Design review of the part built by this model. Coordinates are the model's own, in mm. A direction names the side the tool comes from. Round coordinates to 2 decimals unless told otherwise and drop trailing zeros. Loops run counter-clockwise (first coordinate to the right, second up) from the corner with the lowest first, then second, coordinate; pieces in that order, holes last. Notation, with made-up numbers: M 48,52 L 81,52 A21 ccw 81,74 Z; hole C 63.25,-10.75 d10. An arc over 180 degrees is marked long. One line per item, written item: value. Start each with the question number.
Item 1: For line 1 along Y through (x, z) = (0, 1.3); line 2 along Y through (x, z) = (-8, 1); line 3 along Y through (x, z) = (12.5, 0.7), list the stretches that pass through material, from the lowest coordinate up.
Item 2: For faces 1 (the flat face through (-2.5, 0, 1)), 2 (the flat face through (15, 0, 1)), list the 3-axis set-ups (+Z, -Z, +X, -X, +Y, -Y) from which the entire face can be reached by the end or side of a thin tool; tool diameter is ignored.
Item 3: We need section B-B (x = 8). Write out the cut boundary in (y, z), then the cut area to 3 significant figures.
Item 4: We need section D-D (x = 13). Write out the cut boundary in (y, z), then the cut area to 3 significant figures.
Item 5: We need section A-A (y = -2.5). Write out the cut boundary in (x, z).
Item 6: We need section C-C (z = 1.5). Write out the cut boundary in (x, y).
Item 7: Mouldability with a two-part tool opening along Y and no side actions: class faces 3 (the flat face through (-15, 0, 1)), 4 (the cylindrical face through (11.763, -10.824, 1.014)), 5 (the cylindrical face through (14.1, -13.14, 1.01)) as released by +Y, released by -Y, zero draft, split by the parting line, or undercut.
from build123d import *

# Parameters (mm, degrees)
SKETCH_1_W          = 30
SKETCH_1_H          = 28
EXTRUDE_1_DEPTH     = 2
FILLET_1_R          = 3
SKETCH_2_R          = 1
SKETCH_2_R_2        = 1.25
CUT_EXTRUDE_1_DEPTH = 10
SKETCH_3_R          = 3
CUT_EXTRUDE_2_DEPTH = 10
EXTRUDE_2_DEPTH     = 2


with BuildPart() as part:
    # 草图1 → 凸台-拉伸1 (new body)
    with BuildSketch(Plane.XY):
        Rectangle(SKETCH_1_W, SKETCH_1_H)
    extrude(amount=EXTRUDE_1_DEPTH)

    # 圆角1
    fillet_1_edges = [part.edges().sort_by_distance(p)[0] for p in [
        (-15, -14, 1),
        (-15, 14, 1),
        (15, 14, 1),
        (15, -14, 1),
    ]]
    fillet(fillet_1_edges, radius=FILLET_1_R)

    # 草图2 → 切除-拉伸1 (cut)
    with BuildSketch(Plane.XY.offset(2)):
        with Locations((-12.5, 11.5)):
            Circle(SKETCH_2_R)
        with Locations((12.5, 11.5)):
            Circle(SKETCH_2_R)
        with Locations((-12.5, -11.5)):
            Circle(SKETCH_2_R)
        with Locations((12.5, -11.5)):
            Circle(SKETCH_2_R)
        with Locations((8, 0)):
            Circle(SKETCH_2_R_2)
        with Locations((-8, 0)):
            Circle(SKETCH_2_R_2)
    extrude(amount=-CUT_EXTRUDE_1_DEPTH, mode=Mode.SUBTRACT)

    # 草图3 → 切除-拉伸2 (cut)
    with BuildSketch(Plane.XY.offset(2)):
        Circle(SKETCH_3_R)
    extrude(amount=-CUT_EXTRUDE_2_DEPTH, mode=Mode.SUBTRACT)

    # 草图4 → 凸台-拉伸2 (add)
    with BuildSketch(Plane.XY.offset(2)):
        with BuildLine():
            Line((-2.5, 1.658312395), (-2.5, -1.658312395))
            ThreePointArc((-2.5, -1.658312395), (-3, 0), (-2.5, 1.658312395))
        make_face()
    extrude(amount=-EXTRUDE_2_DEPTH)


solid = part.part
A:
1. line 1: -14 to -3, 3 to 14
1. line 2: -14 to -1.25, 1.25 to 14
1. line 3: -13.96 to -12.5, -10.5 to 10.5, 12.5 to 13.96
2. face 1: +Z, -Z
2. face 2: +Z, -Z, +X, +Y, -Y
3. outline: M -14,0 L -1.25,0 L -1.25,2 L -14,2 Z; M 1.25,0 L 14,0 L 14,2 L 1.25,2 Z
3. area: 51.0 mm2
4. outline: M -13.83,0 L -12.37,0 L -12.37,2 L -13.83,2 Z; M -10.63,0 L 10.63,0 L 10.63,2 L -10.63,2 Z; M 12.37,0 L 13.83,0 L 13.83,2 L 12.37,2 Z
4. area: 48.4 mm2
5. outline: M -15,0 L -1.66,0 L -1.66,2 L -15,2 Z; M 1.66,0 L 15,0 L 15,2 L 1.66,2 Z
6. outline: M -15,-11 A3 ccw -12,-14 L 12,-14 A3 ccw 15,-11 L 15,11 A3 ccw 12,14 L -12,14 A3 ccw -15,11 Z; hole C -12.5,-11.5 d2; hole C -12.5,11.5 d2; hole C -8,0 d2.5; hole M -2.5,-1.66 A3 ccw long -2.5,1.66 Z; hole C 8,0 d2.5; hole C 12.5,-11.5 d2; hole C 12.5,11.5 d2
7. face 3: zero draft
7. face 4: undercut
7. face 5: released by -Y
